Verification items for this drawing (mm, ordinates from the low corner). Round coordinates to 2 decimals unless told otherwise and drop trailing zeros. Write each loop counter-clockwise with the first axis right and the second up, starting at its lowest first coordinate (ties: lowest second). Pieces come first, ordered by that corner, then holes. Notation, with made-up numbers: M 42,35 L 61,35 A22 ccw 61,68 Z; hole C -38.5,-12.5 d8. An arc over 180 degrees is marked long. One line per question, with ' | ' between items. Start each with the question number.
Q1. Cross-section at D-D (x = 82.5). Record the boundary of the cut face in (y, z), then the cut area to 3 significant figures.
Q2. Gauge pin test, flat end, axial feed: pin 1 (24 mm diameter, centred on x = 52.5, y = 81.25, fed in from +Z). Record the tip position at first contact, or that the pin passes through.
Q3. Cross-section at A-A (y = 81.25). State how many separate pieces and enclosed holes the cut face has, then the cut area to 3 significant figures.
Q4. Cross-section at B-B (x = 227.5). Record the boundary of the cut face in (y, z), then the cut area to 3 significant figures.
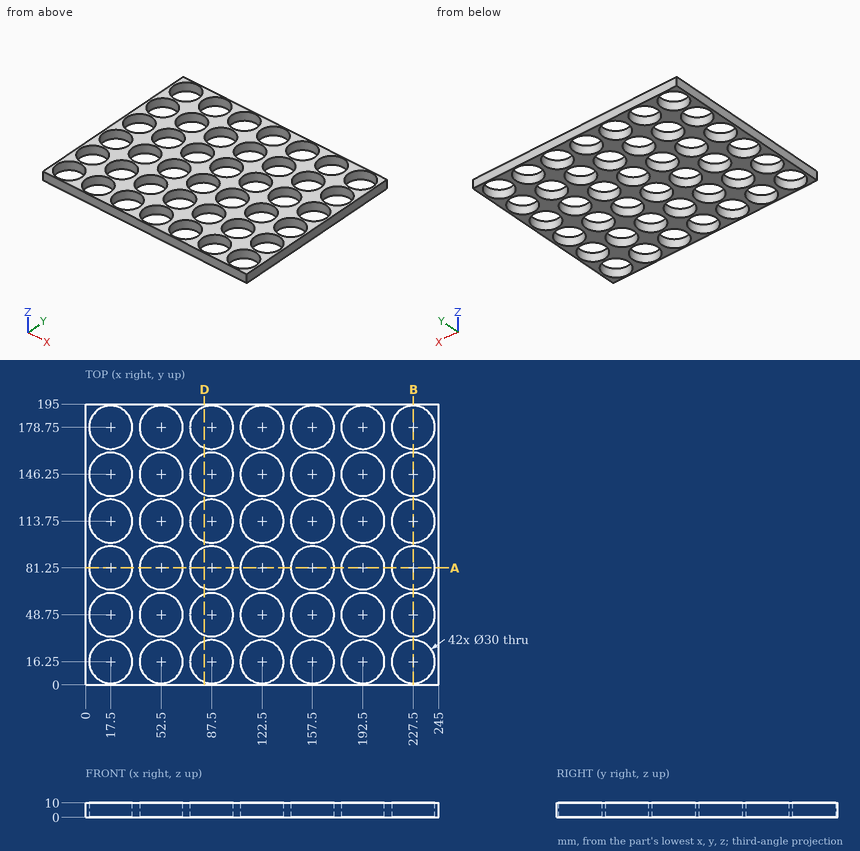
Determined:
1) outline: M 0,0 L 2.11,0 L 2.11,10 L 0,10 Z; M 30.39,0 L 34.61,0 L 34.61,10 L 30.39,10 Z; M 62.89,0 L 67.11,0 L 67.11,10 L 62.89,10 Z; M 95.39,0 L 99.61,0 L 99.61,10 L 95.39,10 Z; M 127.89,0 L 132.11,0 L 132.11,10 L 127.89,10 Z; M 160.39,0 L 164.61,0 L 164.61,10 L 160.39,10 Z; M 192.89,0 L 195,0 L 195,10 L 192.89,10 Z | area: 253 mm²
2) pin 1: passes through
3) separate pieces: 8 | enclosed holes: 0 | area: 350 mm²
4) outline: M 0,0 L 1.25,0 L 1.25,10 L 0,10 Z; M 31.25,0 L 33.75,0 L 33.75,10 L 31.25,10 Z; M 63.75,0 L 66.25,0 L 66.25,10 L 63.75,10 Z; M 96.25,0 L 98.75,0 L 98.75,10 L 96.25,10 Z; M 128.75,0 L 131.25,0 L 131.25,10 L 128.75,10 Z; M 161.25,0 L 163.75,0 L 163.75,10 L 161.25,10 Z; M 193.75,0 L 195,0 L 195,10 L 193.75,10 Z | area: 150 mm²
